Design review of the part built by this model. Coordinates are the model's own, in mm. A direction names the side the tool comes from. Coordinates: 2 decimals unless noted, no trailing zeros. Write each loop counter-clockwise with the first axis right and the second up, starting at its lowest first coordinate (ties: lowest second). Pieces come first, ordered by that corner, then holes.
Q1. Add section D-D, the plane y = -2.75. Give the boundary of the cut face in (x, z), plus the area to 3 significant figures.
Q2. Machinability: for faces 5 (the face through (-22.84, -6, 30)), 6 (the face through (25.65, -6.26, 11.51)), 7 (the face through (54.31, -2.5, 41.95)), which of the approach directions +Z, -Z, +X, -X, +Y, -Y give a long, thin tool a straight path to every point of the face, cutting with its end or side? Answer none if there is none.
Q3. Clearance check with flat-ended pins moving along their axes: pin 1 Ø5 at (y, z) = (-11, 12.5) entering from +X; pin 2 Ø7.5 at (x, y) = (-26.5, -5) entering from -Z; pin 3 Ø1.4 at (y, z) = (-4, 31) entering from -X. State where each tip first meets the part, or that it passes through.
Q4. Add section C-C, the plane z = 26. Give the boundary of the cut face in (x, y).
Q5. The part is to be moulded in two halves that separate along Z. For faces 1 (the face through (51.533, -2.504, 35.253)), 2 (the face through (15.347, -3.131, 24.161)), 3 (the face through (51, -5.08, 40)), 4 (the face through (-26, -6, 31.777)), say which applies: +Z half, -Z half, draft (parallel to the pull), parting line (faces both ways), or undercut.
Q6. To check wall thickness, follow probe 1 along Z at (x, y) = (34, -7); probe 2 along Z at (x, y) = (15, -7); probe 3 along X at (y, z) = (-4.25, 22). State the ranges of each line that lie inside material, in increasing order.
Q7. Add section A-A, the plane y = -7.25. Give the boundary of the cut face in (x, z).
Q8. Add section B-B, the plane x = 20.5. Give the boundary of the cut face in (y, z), plus the area to 3 significant figures.
from build123d import *

# Parameters (mm, degrees)
F1_DEPTH = 12.7
F3_DEPTH = 5.08
F5_DEPTH = 6.35


with BuildPart() as f1:
    # F0 (on Front) → F1 (new body)
    with BuildSketch(Plane.XZ):
        Polygon((23.690905, 22.697873), (27.663032, 0), (55.751652, 0), (49.793456, 35.465427), (44.68644, 40.572446), (-29.649096, 40.572446), (-29.649096, 31.777021), (-22.839734, 31.777021), (-22.839734, 28.939787), (16.030373, 28.939787), align=None)
    extrude(amount=F1_DEPTH)

    # F2 (on Front) → F3 (join)
    with BuildSketch(Plane.XZ):
        Polygon((56.03537, 44.828296), (45.253884, 40.572446), (47.605801, 34.614256), (50.077181, 30.074682), (52.630689, 39.153829), align=None)
    extrude(amount=F3_DEPTH)

    # F4 (on Front) → F5 (join)
    with BuildSketch(Plane.XZ):
        Polygon((23.407178, 23.265319), (17.44899, 27.804894), (13.193138, 20.428086), (15.968651, 18.826828), align=None)
    extrude(amount=F5_DEPTH)


solid = f1.part
Here are the results:
1. outline: (-29.65, 31.78) - (-22.84, 31.78) - (-22.84, 28.94) - (16.03, 28.94) - (17.44, 27.79) - (13.19, 20.43) - (15.97, 18.83) - (23.17, 23.12) - (23.69, 22.7) - (27.66, 0) - (55.75, 0) - (50.47, 31.46) - (52.63, 39.15) - (56.04, 44.83) - (45.25, 40.57) - (45.62, 39.63) - (44.69, 40.57) - (-29.65, 40.57) - close
1. area: 1,820 mm2
2. face 5: -Z, -X, +Y, -Y
2. face 6: -Z, +Y, -Y
2. face 7: +X, +Y, -Y
3. pin 1: stops at x = 54.07
3. pin 2: stops at z = 28.94
3. pin 3: stops at x = -22.84
4. outline: (16.41, -6.35) - (19.64, -6.35) - (19.64, -12.7) - (51.38, -12.7) - (51.38, 0) - (16.41, 0) - close
5. face 1: undercut
5. face 2: undercut
5. face 3: draft
5. face 4: -Z half
6. probe 1: z = 0 to 40.57
6. probe 2: z = 28.94 to 40.57
6. probe 3: x = 14.1 to 21.29, 23.81 to 52.06
7. outline: (-29.65, 31.78) - (-22.84, 31.78) - (-22.84, 28.94) - (16.03, 28.94) - (23.69, 22.7) - (27.66, 0) - (55.75, 0) - (49.79, 35.47) - (44.69, 40.57) - (-29.65, 40.57) - close
8. outline: (-12.7, 25.3) - (-6.35, 25.3) - (-6.35, 21.53) - (0, 21.53) - (0, 40.57) - (-12.7, 40.57) - close
8. area: 218 mm2
